Could you check a few things on this drawing? It's one solid part, dimensions in mm from its lowest x, y, z. Round coordinates to 2 decimals unless told otherwise and drop trailing zeros. Loops run counter-clockwise (first coordinate to the right, second up) from the corner with the lowest first, then second, coordinate; pieces in that order, holes last. Notation, with made-up numbers: M 51.25,11 L 103.25,11 A25 ccw 103.25,26 Z; hole C -28,65.5 d1. An arc over 180 degrees is marked long. Answer as CSV lines item,"result".
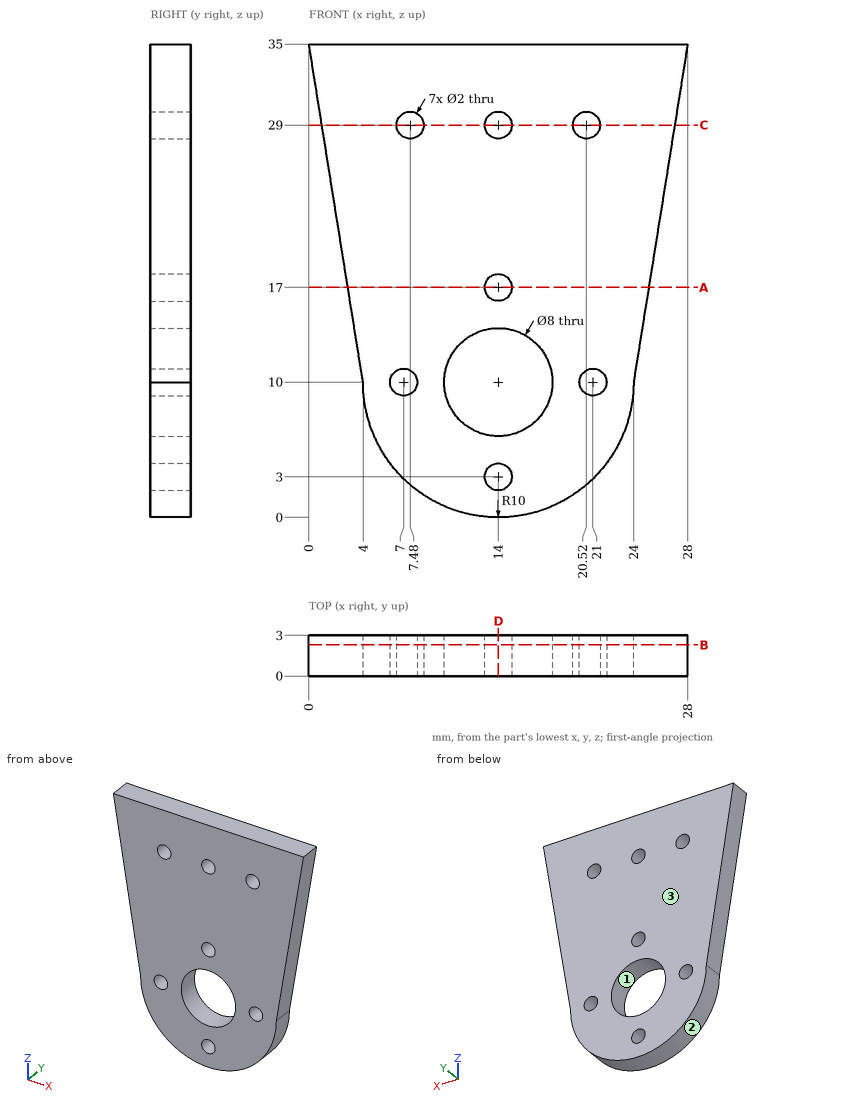
Item 1: If I drill on line 1 along Z through (x, y) = (14, 0.8); line 2 along X through (y, z) = (1.05, 10); line 3 along Z through (x, y) = (21.25, 0.25), over which ranges is the centre line in solid material (lowest first)? Write a range as from..to.
Output:
line 1,"z = 0..2, 4..6, 14..16, 18..28, 30..35"
line 2,"x = 4..6, 8..10, 18..20, 22..24"
line 3,"z = 3.11..9.03, 10.97..28.32, 29.68..35"
Item 2: We'd pull the mould along Z, two halves only. Please class the marked faces 1, 2 and 3: released by +Z, released by -Z, zero draft, split by the parting line, or undercut.
Output:
face 1,"undercut"
face 2,"released by -Z"
face 3,"zero draft"
Item 3: If we section it at C-C on z = 29: Write out the boundary of the cut face in (x, y).
Output:
outline,"M 0.96,0 L 6.48,0 L 6.48,3 L 0.96,3 Z; M 8.48,0 L 13,0 L 13,3 L 8.48,3 Z; M 15,0 L 19.52,0 L 19.52,3 L 15,3 Z; M 21.52,0 L 27.04,0 L 27.04,3 L 21.52,3 Z"
Item 4: If we section it at B-B on y = 2.3: State how many separate pieces and enclosed holes the cut face has, then the cut area to 3 significant figures.
Output:
separate pieces,"1"
enclosed holes,"8"
area,"685 mm2"
Item 5: If we section it at D-D on x = 14: Write out the boundary of the cut face in (y, z), then the cut area to 3 significant figures.
Output:
outline,"M 0,0 L 3,0 L 3,2 L 0,2 Z; M 0,4 L 3,4 L 3,6 L 0,6 Z; M 0,14 L 3,14 L 3,16 L 0,16 Z; M 0,18 L 3,18 L 3,28 L 0,28 Z; M 0,30 L 3,30 L 3,35 L 0,35 Z"
area,"63.0 mm2"
Item 6: If we section it at A-A on z = 17: Write out the boundary of the cut face in (x, y), then the cut area to 3 significant figures.
Output:
outline,"M 2.88,0 L 13,0 L 13,3 L 2.88,3 Z; M 15,0 L 25.12,0 L 25.12,3 L 15,3 Z"
area,"60.7 mm2"
